```python
from build123d import *

# Parameters (mm, degrees)
SKETCH_1_R                 = 18.65
EXTRUDE_1_DEPTH            = 2
SKETCH_2_R                 = 1.55
CUT_EXTRUDE_1_DEPTH        = 2
HOLE_WIZARD_M21_AT_2_COUNT = 2
HOLE_WIZARD_M21_AT_2_PITCH = 32.3


with BuildPart() as part:
    # Эскиз1 → Бобышка-Вытянуть1 (new body)
    with BuildSketch(Plane(origin=(0, 0, 0), x_dir=(1, 0, 0), z_dir=(0, 1, 0))):
        Circle(SKETCH_1_R)
    extrude(amount=EXTRUDE_1_DEPTH)

    # Эскиз2 → Вырез-Вытянуть1 (cut)
    with BuildSketch(Plane(origin=(0, 2, 0), x_dir=(1, 0, 0), z_dir=(0, 1, 0))):
        with Locations((7, 0)):
            Circle(SKETCH_2_R)
    extrude(amount=-CUT_EXTRUDE_1_DEPTH, mode=Mode.SUBTRACT)

    # Эскиз4 → Зенковка для  винта с плоской головкой M21 (revolve, cut)
    with BuildSketch(Plane(origin=(0, 2, -16.15), x_dir=(0, 0, 1), z_dir=(1, 0, 0))):
        Polygon((0, 0), (0, 2), (1.2, 2), (1.2, 1), (2.2, 0), align=None)
    hole_wizard_m21 = revolve(axis=Axis((0, 8.35, -16.15), (0, -1, 0)), mode=Mode.SUBTRACT)

    # Зенковка для  винта с плоской головкой M21 at 2: Зенковка для  винта с плоской головкой M21 ×2
    with Locations(*[(0, 0, i * HOLE_WIZARD_M21_AT_2_PITCH) for i in range(1, HOLE_WIZARD_M21_AT_2_COUNT)]):
        add(hole_wizard_m21, mode=Mode.SUBTRACT)


solid = part.part
```
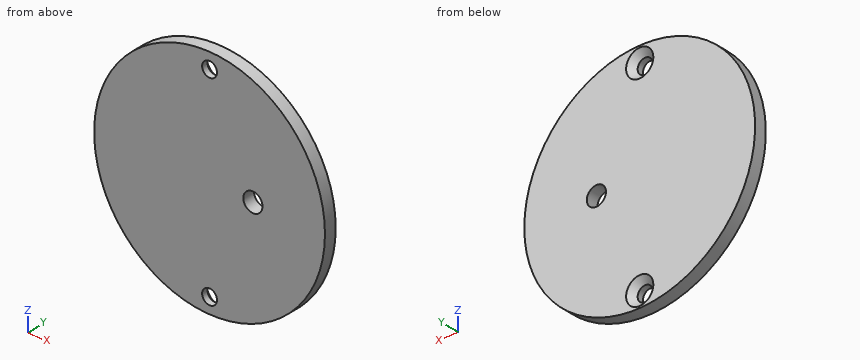
For this review, take the finished solid that the model builds, in its own axes (mm). Round coordinates to 2 decimals unless told otherwise and drop trailing zeros. Write each loop counter-clockwise with the first axis right and the second up, starting at its lowest first coordinate (ties: lowest second). Pieces come first, ordered by that corner, then holes.
1) Take a section at C-C on y = 1.45. Give the boundary of the cut face in (x, z).
Answer below:
outline: circle Ø37.3 at (0, 0); hole circle Ø3.3 at (0, -16.15); hole circle Ø3.3 at (0, 16.15); hole circle Ø3.1 at (7, 0)
2) Take a section at B-B on z = 0. Give the boundary of the cut face in (x, y).
Answer below:
outline: (-18.65, 0) - (5.45, 0) - (5.45, 2) - (-18.65, 2) - close; (8.55, 0) - (18.65, 0) - (18.65, 2) - (8.55, 2) - close
3) Take a section at A-A on x = 0. Give the boundary of the cut face in (y, z), then the cut area to 3 significant figures.
Answer below:
outline: (0, -18.65) - (2, -18.65) - (2, -18.35) - (1, -17.35) - (0, -17.35) - close; (0, -14.95) - (1, -14.95) - (2, -13.95) - (2, 13.95) - (1, 14.95) - (0, 14.95) - close; (0, 17.35) - (1, 17.35) - (2, 18.35) - (2, 18.65) - (0, 18.65) - close
area: 63.0 mm2
4) For line 1 along Z through (x, y) = (0, 0.55); line 2 along X through (y, z) = (0.9, 0); line 3 along Z through (x, y) = (-0.5, 0.75), list the stretches that pass through material, from the lowest coordinate up.
Answer below:
line 1: z = -18.65 to -17.35, -14.95 to 14.95, 17.35 to 18.65
line 2: x = -18.65 to 5.45, 8.55 to 18.65
line 3: z = -18.64 to -17.24, -15.06 to 15.06, 17.24 to 18.64
5) Insertion check: pin 1 Ø1 at (x, y) = (-3, 0.5) entering from +Z. The pin has a flat end and moves straight along its axis. Give the tip position at first contact, or say it passes through.
Answer below:
pin 1: stops at z = 18.48
6) Take a section at D-D on x = 7.5. Give the boundary of the cut face in (y, z).
Answer below:
outline: (0, -17.08) - (2, -17.08) - (2, -1.47) - (0, -1.47) - close; (0, 1.47) - (2, 1.47) - (2, 17.08) - (0, 17.08) - close
